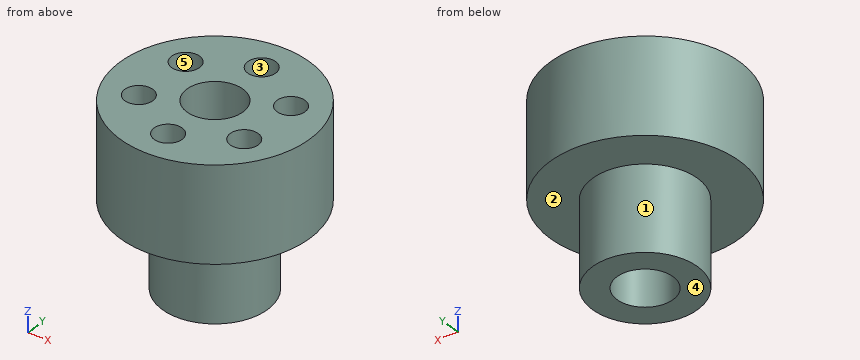
Autodesk Inventor part; units mm, degrees
ref_plane "YZ Plane" through (0, 0, 0) normal (1, 0, 0) x (0, 1, 0)
ref_plane "XZ Plane" through (0, 0, 0) normal (0, 1, 0) x (-1, 0, 0)
ref_plane "XY Plane" through (0, 0, 0) normal (0, 0, 1) x (1, 0, 0)
sketch "Szkic1" plane through (0, 0, 0) normal (0, 0, 1) x (1, 0, 0)
  circle A0 centre (0, 0) radius 13.5
  dimension "d0" = 27
extrude "Wyciągnięcie proste1" add sketch "Szkic1" along normal blind 25.5
sketch "Szkic2" plane through (0, 0, 0) normal (0, 0, -1) x (-1, 0, 0)
  circle A0 centre (0, 0) radius 7.5
  circle A1 centre (0, 0) radius 13.5
  dimension "d3" = 15
extrude "Wyciągnięcie proste2" cut sketch "Szkic2" against normal blind 12
sketch "Szkic3" plane through (0, 0, 0) normal (0, 0, -1) x (-1, 0, 0)
  circle A0 centre (0, 0) radius 4
  dimension "d6" = 8
extrude "Wyciągnięcie proste3" cut sketch "Szkic3" against normal up to next
sketch "Szkic4" plane through (0, 0, 25.5) normal (0, 0, 1) x (1, 0, 0)
  circle A0 centre (0, 0) radius 4
  circle A1 centre (0, 0) radius 13.5
  line L0 (0, 0) -> (0, 8.75)
  circle A2 centre (0, 8.75) radius 2
  dimension "d11" = 8.75
  dimension "d12" = 4
extrude "Wyciągnięcie proste4" cut sketch "Szkic4" against normal blind 12 contours A2
pattern_circular "Szyk kołowy1" count 6 over 360 about axis through (0, 0, 0) along (0, 0, 1) of "Wyciągnięcie proste4"
thread "Gwint1"
thread "Gwint2"
thread "Gwint3"
thread "Gwint4"
thread "Gwint5"
thread "Gwint6"
properties part number "Tuleja zaciskowo rozprężna RCK BK 80 8x15 Clampex"
For this review, take the finished solid that the model builds, in its own axes (mm). Face numbers are marked on the shaded views. A direction names the side the tool comes from. Give positions to 0.01 mm unless a question says otherwise; leave off trailing zeros. Write each loop counter-clockwise with the first axis right and the second up, starting at its lowest first coordinate (ties: lowest second). Pieces come first, ordered by that corner, then holes.
Item 1: Take a section at A-A (x = 0). Give the boundary of the cut face in (y, z), and give its area (4 significant figures).
Item 2: Take a section at C-C (z = 4). Give the boundary of the cut face in (x, y), and give its area (3 significant figures).
Item 3: Insertion check: P1, Ø1, axis at x = 9.5, z = 13, coming from the -Y side; P2, Ø5, axis at x = 10.5, z = 16.5, coming from the +Y side; P3, Ø2, axis at x = 0.5, y = 8.5, coming from the +Z side. Each pin has a flat end and moves straight along its axis. Give the tip position at first contact, or say it passes through.
Item 4: Take a section at D-D (z = 22.5). Give the boundary of the cut face in (x, y) (3 decimals).
Item 5: Take a section at B-B (y = 0). Give the boundary of the cut face in (x, z).
Item 6: Machinability: for the marked faces 4 and 5, which of the approach directions +Z, -Z, +X, -X, +Y, -Y give a long, thin tool a straight path to every point of the face, cutting with its end or side? Answer none if there is none.
Item 7: The part is to be moulded in two halves that separate along Y. For the marked faces 1, 2 and 3, say which applies: +Y half, -Y half, draft (parallel to the pull), parting line (faces both ways), or undercut.
Item 8: Wall thickness on probe 1 along Y at (x, z) = (0, 20); probe 2 along Y at (x, z) = (-8.75, 22.25); probe 3 along Y at (x, z) = (0, 10.5): over which ranges is each line inside the solid? List them lowest first.
Established:
1. outline: (-13.5, 12) - (-7.5, 12) - (-7.5, 0) - (-4, 0) - (-4, 25.5) - (-6.75, 25.5) - (-6.75, 13.5) - (-10.75, 13.5) - (-10.75, 25.5) - (-13.5, 25.5) - close; (4, 0) - (7.5, 0) - (7.5, 12) - (13.5, 12) - (13.5, 25.5) - (10.75, 25.5) - (10.75, 13.5) - (6.75, 13.5) - (6.75, 25.5) - (4, 25.5) - close
1. area: 244.5 mm2
2. outline: circle Ø15 at (0, 0); hole circle Ø8 at (0, 0)
2. area: 126 mm2
3. P1: stops at y = -10.06
3. P2: stops at y = 10.87
3. P3: stops at z = 13.5
4. outline: circle Ø27 at (0, 0); hole circle Ø4 at (-7.578, -4.375); hole circle Ø4 at (-7.578, 4.375); hole circle Ø8 at (0, 0); hole circle Ø4 at (0, -8.75); hole circle Ø4 at (0, 8.75); hole circle Ø4 at (7.578, -4.375); hole circle Ø4 at (7.578, 4.375)
5. outline: (-13.5, 12) - (-7.5, 12) - (-7.5, 0) - (-4, 0) - (-4, 25.5) - (-13.5, 25.5) - close; (4, 0) - (7.5, 0) - (7.5, 12) - (13.5, 12) - (13.5, 25.5) - (4, 25.5) - close
6. face 4: -Z, +X, -X, +Y, -Y
6. face 5: +Z
7. face 1: parting line
7. face 2: draft
7. face 3: undercut
8. probe 1: y = -13.5 to -10.75, -6.75 to -4, 4 to 6.75, 10.75 to 13.5
8. probe 2: y = -10.28 to -6, -2.75 to 2.75, 6 to 10.28
8. probe 3: y = -7.5 to -4, 4 to 7.5
